Build history of the part. All positions in model axes, mm. Face numbers are marked on the shaded views. A direction names the side the tool comes from. Coordinates: 2 decimals unless noted, no trailing zeros. Order: outer loops, then holes, each group sorted by start corner. A loop starts at its lowest first (then second) coordinate and runs counter-clockwise, first axis right, second up. Notation, with made-up numbers: (64, -9.5) - (96, -9.5) arc R32 ccw to (96, 28.5) - close; hole circle Ø8 at (28, 24). An arc over 180 degrees is marked (long way). Write each question's results on one line, items separated by ' | '. Start each with the question number.
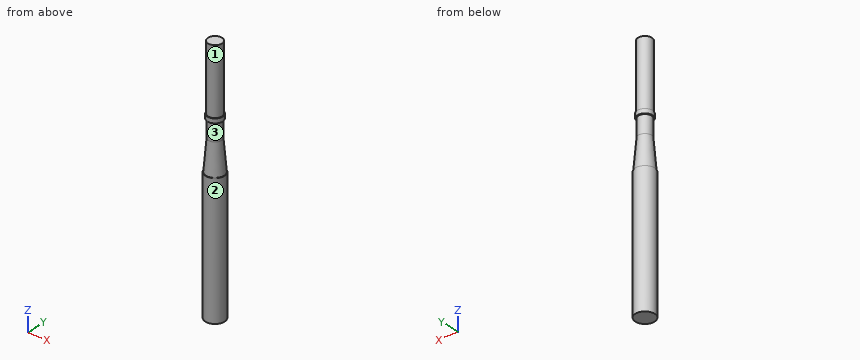
Autodesk Inventor part; units mm, degrees
ref_plane "Work Plane1" through (0, 0, -120) normal (0, 0, -1) x (-1, 0, 0)
ref_plane "YZ Plane" through (0, 0, 0) normal (1, 0, 0) x (0, 1, 0)
ref_plane "XZ Plane" through (0, 0, 0) normal (0, 1, 0) x (-1, 0, 0)
sketch "Sketch1" plane through (0, 0, 0) normal (0, 0, 1) x (1, 0, 0)
  circle A0 centre (0, 0) radius 16
  dimension "d0" = 32
extrude "Extrusion1" add sketch "Sketch1" along normal blind 150
sketch "Sketch2" plane through (0, 0, 0) normal (0, 0, -1) x (-1, 0, 0)
  circle A0 centre (0, 0) radius 17.5
  dimension "d3" = 35
extrude "Extrusion2" add sketch "Sketch2" along normal blind 10
sketch "Sketch3" plane through (0, 0, -10) normal (0, 0, -1) x (-1, 0, 0)
  circle A0 centre (0, 0) radius 15
  dimension "d6" = 30
extrude "Extrusion3" add sketch "Sketch3" along normal blind 40
sketch "Sketch4" plane through (0, 0, -50) normal (0, 0, -1) x (-1, 0, 0)
  circle A0 centre (0, 0) radius 15
  dimension "d10" = 30
ref_plane "Work Plane1" through (0, 0, -120) normal (0, 0, -1) x (-1, 0, 0)
sketch "Sketch5" plane through (0, 0, -120) normal (0, 0, -1) x (-1, 0, 0)
  circle A0 centre (0, 0) radius 16
  circle A1 centre (0, 0) radius 21
  dimension "d11" = 42
loft "Loft1" add profiles "Sketch5" section 1 edges at (15, 0, -50) contours A0 | A1
sketch "Sketch6" plane through (0, 0, -120) normal (0, 0, -1) x (-1, 0, 0)
  circle A0 centre (0, 0) radius 22
  dimension "d16" = 44
extrude "Extrusion4" add sketch "Sketch6" along normal blind 300
properties part number "oar"
Item 1: Which spindle directions (+Z, -Z, +X, -X, +Y, -Y) get a long thin tool onto all of the face, cutting with end or side? Do the marked faces 1, 2 and 3. Say none if no direction does.
Item 2: Slice it at C-C (z = -41.5). Write the cut outline in (x, y).
Item 3: Flat gauge pins, fed straight in: P1, Ø2, axis at x = -11.5, z = -320, coming from the -Y side; P2, Ø10, axis at x = -8.5, z = -109.5, coming from the +Y side; P3, Ø1.5, axis at x = -6.5, z = -250.5, coming from the -Y side. Where does each tip first touch, or does it go through?
Item 4: Slice it at B-B (z = 82.5). Write the cut outline in (x, y), then the cut area to 3 significant figures.
Item 5: Slice it at A-A (x = 0). Write the cut outline in (y, z), then the cut area to 3 significant figures.
Item 6: Probe probe 1 along X at (y, z) = (-0.5, 33); probe 2 along X at (y, z) = (2, -260.5); probe 3 along Z at (x, y) = (11, 18). List the from-to ranges inside material, lowest first.
Resolved:
1) face 1: +Z | face 2: +Z, -Z | face 3: none
2) outline: circle Ø30 at (0, 0)
3) P1: y = -19.33 | P2: y = 19.89 | P3: y = -21.24
4) outline: circle Ø32 at (0, 0) | area: 804 mm^2
5) outline: (-22, -420) - (22, -420) - (22, -120) - (21, -120) - (15, -50) - (15, -10) - (17.5, -10) - (17.5, 0) - (16, 0) - (16, 150) - (-16, 150) - (-16, 0) - (-17.5, 0) - (-17.5, -10) - (-15, -10) - (-15, -50) - (-21, -120) - (-22, -120) - close | area: 22,100 mm^2
6) probe 1: -15.99 to 15.99 | probe 2: -21.91 to 21.91 | probe 3: -420 to -120
